Build history of the part. All positions in model axes, mm. Face numbers are marked on the shaded views. A direction names the side the tool comes from. Give positions to 0.01 mm unless a question says otherwise; leave off trailing zeros. Order: outer loops, then holes, each group sorted by start corner. A loop starts at its lowest first (then second) coordinate and runs counter-clockwise, first axis right, second up. Notation, with made-up numbers: (-39, 50.5) - (-17, 50.5) arc R14 ccw to (-17, 72.5) - close; hole circle Ø2 at (-3, 78). An arc over 180 degrees is marked (long way). Use a Markdown table: item, result.
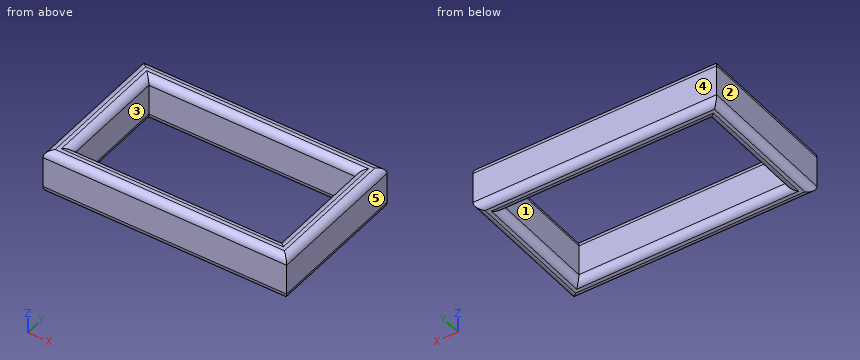
from build123d import *

# Parameters (mm, degrees)
F0_W     = 27
F0_H     = 16
F0_W_2   = 23
F0_H_2   = 12
F1_DEPTH = 5
F2_R     = 0.8


with BuildPart() as f1:
    # F0 (on Top) → F1 (new body)
    with BuildSketch(Plane.XY):
        Rectangle(F0_W, F0_H)
        Rectangle(F0_W_2, F0_H_2, mode=Mode.SUBTRACT)
    extrude(amount=F1_DEPTH)

    # F2
    f2_edges = [f1.edges().sort_by_distance(p)[0] for p in [
        (0, 8, 5),
        (13.5, 0, 5),
        (0, -8, 5),
        (-13.5, 0, 5),
        (-11.5, 0, 5),
        (0, 6, 5),
        (0, -6, 5),
        (11.5, 0, 5),
        (0, -8, 0),
        (0, -6, 0),
        (0, 6, 0),
        (0, 8, 0),
        (13.5, 0, 0),
        (11.5, 0, 0),
        (-13.5, 0, 0),
        (-11.5, 0, 0),
    ]]
    fillet(f2_edges, radius=F2_R)


solid = f1.part
1) Slice it at C-C (z = 2.95). Write the cut outline in (x, y), and give its area (3 significant figures).
Computed:
| item | result |
|---|---|
| outline | (-13.5, -8) - (13.5, -8) - (13.5, 8) - (-13.5, 8) - close; hole (-11.5, -6) - (11.5, -6) - (11.5, 6) - (-11.5, 6) - close |
| area | 156 mm² |
2) Slice it at B-B (x = 1.5). Write the cut outline in (y, z).
Computed:
| item | result |
|---|---|
| outline | (-8, 0.8) arc R0.8 ccw to (-7.2, 0) - (-6.8, 0) arc R0.8 ccw to (-6, 0.8) - (-6, 4.2) arc R0.8 ccw to (-6.8, 5) - (-7.2, 5) arc R0.8 ccw to (-8, 4.2) - close; (6, 0.8) arc R0.8 ccw to (6.8, 0) - (7.2, 0) arc R0.8 ccw to (8, 0.8) - (8, 4.2) arc R0.8 ccw to (7.2, 5) - (6.8, 5) arc R0.8 ccw to (6, 4.2) - close |
3) Two-plate mould, pull along X, no slides. Class the marked faces 3, 4 and 5: +X half, -X half, draft (parallel to the pull), parting line (faces both ways), or undercut.
Computed:
| item | result |
|---|---|
| face 3 | undercut |
| face 4 | draft |
| face 5 | +X half |
4) Wall check: line 1 (Y direction, x = -9, z = 2.7); line 2 (X direction, y = 2.5, z = 3.4); line 3 (X direction, y = -5.5, z = 4.8). Give the ranges that are in metal, low to high. Write a range as from..to.
Computed:
| item | result |
|---|---|
| line 1 | y = -8..-6, 6..8 |
| line 2 | x = -13.5..-11.5, 11.5..13.5 |
| line 3 | x = -13.23..-11.77, 11.77..13.23 |
5) Slice it at D-D (y = 6.5). Write the cut outline in (x, z).
Computed:
| item | result |
|---|---|
| outline | (-13.5, 0.8) arc R0.8 ccw to (-12.7, 0) - (-12.3, 0) arc R0.8 ccw to (-12, 0.06) - (12, 0.06) arc R0.8 ccw to (12.3, 0) - (12.7, 0) arc R0.8 ccw to (13.5, 0.8) - (13.5, 4.2) arc R0.8 ccw to (12.7, 5) - (12.3, 5) arc R0.8 ccw to (12, 4.94) - (-12, 4.94) arc R0.8 ccw to (-12.3, 5) - (-12.7, 5) arc R0.8 ccw to (-13.5, 4.2) - close |
6) Tool access for the marked faces 1 and 2: list every direction of +Z, -Z, +X, -X, +Y, -Y with a clear straight run to the whole face (end or side of a thin tool).
Computed:
| item | result |
|---|---|
| face 1 | +Z, -Z |
| face 2 | +Z, -Z, -X, +Y, -Y |
7) Slice it at A-A (y = 1). Write the cut outline in (x, z), and give its area (3 significant figures).
Computed:
| item | result |
|---|---|
| outline | (-13.5, 0.8) arc R0.8 ccw to (-12.7, 0) - (-12.3, 0) arc R0.8 ccw to (-11.5, 0.8) - (-11.5, 4.2) arc R0.8 ccw to (-12.3, 5) - (-12.7, 5) arc R0.8 ccw to (-13.5, 4.2) - close; (11.5, 0.8) arc R0.8 ccw to (12.3, 0) - (12.7, 0) arc R0.8 ccw to (13.5, 0.8) - (13.5, 4.2) arc R0.8 ccw to (12.7, 5) - (12.3, 5) arc R0.8 ccw to (11.5, 4.2) - close |
| area | 18.9 mm² |
